Read the model definition and answer for the solid it produces. Units are mm, in the model's axes. A direction names the side the tool comes from. Round coordinates to 2 decimals unless told otherwise and drop trailing zeros. Loops run counter-clockwise (first coordinate to the right, second up) from the corner with the lowest first, then second, coordinate; pieces in that order, holes last. Notation, with made-up numbers: (-3.75, 6.5) - (26.25, 6.5) arc R22 ccw to (26.25, 29.5) - close; hole circle Ø6 at (18.5, 42.25). An arc over 180 degrees is marked (long way). Answer as CSV lines item,"result".
```python
from build123d import *

# Parameters (mm, degrees)
SKETCH_1_R           = 21.25
EXTRUDE_1_DEPTH      = 51.5
SKETCH_2_R           = 1.5
EXTRUDE_2_DEPTH      = 4
SKETCH_3_R           = 8.75
CUT_EXTRUDE_1_DEPTH  = 1.5
SKETCH_4_R           = 2.5
CUT_EXTRUDE_2_DEPTH  = 6.3
SKETCH_5_R           = 2
CUT_EXTRUDE_3_DEPTH  = 7
SKETCH_7_R           = 12.5
EXTRUDE_3_DEPTH      = 2.5
SKETCH_11_R          = 4
EXTRUDE_5_DEPTH      = 25
CUT_EXTRUDE_11_DEPTH = 3.5
SKETCH_13_R          = 2
CUT_EXTRUDE_10_DEPTH = 7


with BuildPart() as part:
    # 草圖1 → 填料-伸長1 (new body)
    with BuildSketch(Plane.XY):
        Circle(SKETCH_1_R)
    extrude(amount=EXTRUDE_1_DEPTH)

    # 草圖2 → 填料-伸長2 (add)
    with BuildSketch(Plane(origin=(0, 0, 0), x_dir=(-1, 0, 0), z_dir=(0, 0, -1))):
        with Locations((0, 12.5)):
            Circle(SKETCH_2_R)
        with Locations((0, -12.5)):
            Circle(SKETCH_2_R)
    extrude(amount=EXTRUDE_2_DEPTH)

    # 草圖3 → 除料-伸長1 (cut)
    with BuildSketch(Plane(origin=(0, 0, 0), x_dir=(-1, 0, 0), z_dir=(0, 0, -1))):
        Circle(SKETCH_3_R)
    extrude(amount=-CUT_EXTRUDE_1_DEPTH, mode=Mode.SUBTRACT)

    # 草圖4 → 除料-伸長2 (cut)
    with BuildSketch(Plane(origin=(0, 0, 1.5), x_dir=(-1, 0, 0), z_dir=(0, 0, -1))):
        Circle(SKETCH_4_R)
    extrude(amount=-CUT_EXTRUDE_2_DEPTH, mode=Mode.SUBTRACT)

    # 草圖5 → 除料-伸長3 (cut)
    with BuildSketch(Plane(origin=(0, 0, 7.8), x_dir=(-1, 0, 0), z_dir=(0, 0, -1))):
        Circle(SKETCH_5_R)
    extrude(amount=-CUT_EXTRUDE_3_DEPTH, mode=Mode.SUBTRACT)

    # 草圖7 → 填料-伸長3 (add)
    with BuildSketch(Plane.XY.offset(51.5)):
        Circle(SKETCH_7_R)
    extrude(amount=EXTRUDE_3_DEPTH)

    # 草圖11 → 填料-伸長5 (add)
    with BuildSketch(Plane.XY.offset(54)):
        Circle(SKETCH_11_R)
    extrude(amount=EXTRUDE_5_DEPTH)

    # 草圖12 → 除料-伸長11 (cut)
    with BuildSketch(Plane(origin=(0, -4, 0), x_dir=(1, 0, 0), z_dir=(0, 1, 0))):
        with BuildLine():
            Line((-1.65, -74.85), (-1.65, -58.15))
            ThreePointArc((-1.65, -58.15), (0, -56.5), (1.65, -58.15))
            Line((1.65, -58.15), (1.65, -74.85))
            ThreePointArc((1.65, -74.85), (0, -76.5), (-1.65, -74.85))
        make_face()
    extrude(amount=CUT_EXTRUDE_11_DEPTH, mode=Mode.SUBTRACT)

    # 草圖13 → 除料-伸長10 (cut)
    with BuildSketch(Plane.XY.offset(51.5)):
        with Locations((16, 0)):
            Circle(SKETCH_13_R)
        with Locations((0, -16)):
            Circle(SKETCH_13_R)
        with Locations((-16, 0)):
            Circle(SKETCH_13_R)
        with Locations((0, 16)):
            Circle(SKETCH_13_R)
        with Locations((11.313708499, 11.313708499)):
            Circle(SKETCH_13_R)
        with Locations((11.313708499, -11.313708499)):
            Circle(SKETCH_13_R)
        with Locations((-11.313708499, -11.313708499)):
            Circle(SKETCH_13_R)
        with Locations((-11.313708499, 11.313708499)):
            Circle(SKETCH_13_R)
    extrude(amount=-CUT_EXTRUDE_10_DEPTH, mode=Mode.SUBTRACT)


solid = part.part
```
1) Find the intervals of material crossed by line 1 (Y direction, x = 0, z = 46); line 2 (Z direction, x = 8, y = -18); line 3 (Z direction, x = -4.5, y = 5), in increasing order.
Entries:
line 1,"y = -21.25 to -18, -14 to 14, 18 to 21.25"
line 2,"z = 0 to 51.5"
line 3,"z = 1.5 to 54"
2) Each of these flat-tipped pins is pushed along its axis until it touches: P1, Ø4.5, axis at x = -15, y = -1, coming from the +Z side; P2, Ø2.5, axis at x = 0, y = -16, coming from the -Z side; P3, Ø2, axis at x = -1, y = 1, coming from the -Z side. Where does it stop, or does it pass through?
Entries:
P1,"stops at z = 51.5"
P2,"stops at z = 0"
P3,"stops at z = 7.8"
3) A cutting plane is placed at D-D, the plane x = 11.5. Determine the outline of the cut face in (y, z).
Entries:
outline,"(-17.87, 0) - (17.87, 0) - (17.87, 51.5) - (13.31, 51.5) - (13.31, 44.5) - (9.32, 44.5) - (9.32, 51.5) - (4.9, 51.5) - (4.9, 54) - (-4.9, 54) - (-4.9, 51.5) - (-9.32, 51.5) - (-9.32, 44.5) - (-13.31, 44.5) - (-13.31, 51.5) - (-17.87, 51.5) - close"
4) The mould has two halves that part along Z. Classify faces 4 (the face through (0, 16, 44.5)), 5 (the face through (14.4, -1.2, 48)), 6 (the face through (0, -2.3, 76.5)), 7 (the face through (0, 0, 14.8)): pulls with the +Z half, pulls with the -Z half, needs draft (parallel to the pull), parting line crosses it, or undercut.
Entries:
face 4,"pulls with the +Z half"
face 5,"needs draft"
face 6,"undercut"
face 7,"pulls with the -Z half"
5) A cutting plane is placed at B-B, the plane x = -17. Determine the outline of the cut face in (y, z), plus the area to 3 significant figures.
Entries:
outline,"(-12.75, 0) - (12.75, 0) - (12.75, 51.5) - (1.73, 51.5) - (1.73, 44.5) - (-1.73, 44.5) - (-1.73, 51.5) - (-12.75, 51.5) - close"
area,"1,290 mm^2"
6) A cutting plane is placed at C-C, the plane z = 20. Determine the outline of the cut face in (x, y).
Entries:
outline,"circle Ø42.5 at (0, 0)"
7) A tool of negligible diameter and unlimited length cuts with its end or side. For faces 1 (the face through (0, -12, -4)), 2 (the face through (0, -0.5, 66)), 3 (the face through (16, 0, 44.5)), from which of +Z, -Z, +X, -X, +Y, -Y can it reach the whole face along a straight path? Write none if from no direction.
Entries:
face 1,"-Z, +X, -X, +Y, -Y"
face 2,"-Y"
face 3,"+Z"
